Autodesk Inventor part; units mm, degrees
ref_plane "YZ Plane" through (0, 0, 0) normal (1, 0, 0) x (0, 1, 0)
ref_plane "XZ Plane" through (0, 0, 0) normal (0, 1, 0) x (-1, 0, 0)
ref_plane "XY Plane" through (0, 0, 0) normal (0, 0, 1) x (1, 0, 0)
sketch "Skizze3" plane through (0, 0, 0) normal (0, 1, 0) x (-1, 0, 0)
  line L0 (0, 0) -> (0, -150) construction
  line L1 (-10, 0) -> (-10, -150)
  line L2 (10, -150) -> (10, 0)
  arc A0 (10, 0) -> (-10, 0) centre (0, 0) ccw
  arc A1 (-10, -150) -> (10, -150) centre (0, -150) ccw
  circle A2 centre (0, 0) radius 5
  circle A3 centre (0, -150) radius 2.5
  circle A4 centre (0, -140) radius 1.5
  circle A5 centre (0, -115) radius 5
  circle A6 centre (0, -100) radius 5
  circle A7 centre (0, 0) radius 4.5
  circle A8 centre (0, -85) radius 5
  point P0 (0, -75)
  dimension "d4" = 150
  dimension "d5" = 10
  dimension "d6" = 10
  dimension "d7" = 5
  dimension "d8" = 3
  dimension "d9" = 10
  dimension "d12" = 10
  dimension "d13" = 10
  dimension "d15" = 15
  dimension "d27" = 9
  dimension "d34" = 115
  dimension "d35" = 15
extrude "Extrusion3" add sketch "Skizze3" along normal blind 5 contours A0 L2 A1 L1
sketch "Skizze4" plane through (0, 5, 0) normal (0, 1, 0) x (1, 0, 0)
  circle A0 centre (0, 0) radius 5
  circle A1 centre (0, 0) radius 10
  dimension "d18" = 20
extrude "Extrusion4" add sketch "Skizze4" along normal blind 5
extrude "Extrusion5" add sketch "Skizze3" along normal blind 6 contours A2
sketch "Skizze5" plane through (0, 0, 0) normal (0, -1, 0) x (1, 0, 0)
  circle A0 centre (0, -130) radius 5
  circle A1 centre (0, -100) radius 5
  circle A2 centre (0, -115) radius 5
  circle A3 centre (0, -100) radius 4.5
  circle A4 centre (0, -115) radius 4.5
  circle A5 centre (0, -130) radius 4.5
  point P0 (0, 0)
  point P1 (-1.5, -140)
  point P2 (-1.5, -140)
  dimension "d28" = 9
  dimension "d29" = 9
  dimension "d30" = 9
extrude "Extrusion7" add sketch "Skizze5" against normal blind 1 contours A1 | A2
equation "\"d4\" = Gelenk_Stifthalter"
equation "\"d35\" = d15"
equation "\"Gelenk_Stifthalter\" = 150"
properties part number "BT303_trajan20_21" material "Kunststoff, undurchsichtig Schwarz"
Can you work these out from the model? Positions are in its coordinate system, mm. A direction names the side the tool comes from. Give positions to 0.01 mm unless a question says otherwise; leave off trailing zeros. Order: outer loops, then holes, each group sorted by start corner. A loop starts at its lowest first (then second) coordinate and runs counter-clockwise, first axis right, second up. Notation, with made-up numbers: M 73.5,-7 L 131.5,-7 A22 cw 131.5,13 Z; hole C -7.75,-3 d10. An arc over 180 degrees is marked long. One line per item, written item: value.
Item 1: If we mould it in two halves opening along Z, with no side actions, what happens to faces 1 (the face through (0.195, 2.465, -141.487)), 2 (the face through (0, 2, -160)), 3 (the face through (10, 2, -74))? For each: pulls with the +Z half, pulls with the -Z half, needs draft (parallel to the pull), parting line crosses it, or undercut.
Verdict:
face 1: undercut
face 2: pulls with the -Z half
face 3: needs draft
Item 2: Please list where these lines run through material, in increasing order: line 1 (Z direction, x = -4, y = 2.5); line 2 (Z direction, x = 3, y = 1.75); line 3 (X direction, y = 3.2, z = -100).
Verdict:
line 1: -159.17 to -118, -112 to -103, -97 to -88, -82 to -2.06, 2.06 to 9.17
line 2: -159.54 to -119, -111 to -104, -96 to -89, -81 to -3.35, 3.35 to 9.54
line 3: -10 to -5, 5 to 10
Item 3: If we section it at B-B on y = 3: Write out the boundary of the cut face in (x, z).
Verdict:
outline: M -10,-150 A10 ccw 10,-150 L 10,0 A10 ccw -10,0 Z; hole C 0,-115 d10; hole C 0,-100 d10; hole C 0,-85 d10; hole C 0,0 d9; hole C 0,-150 d5; hole C 0,-140 d3
Item 4: For pin 1 (5 mm diameter, centred on x = -1, z = 2, fed in from +Y); pin 2 (11 mm diameter, centred on x = 2, z = -97.5, fed in from +Y), each with a flat end and sliding along its axis, tell me the tip position at first contact or that it passes through.
Verdict:
pin 1: y = 6
pin 2: y = 5
Item 5: If we section it at C-C on x = 0: State how many separate pieces and enclosed holes the cut face has, and give its area (3 significant figures).
Verdict:
separate pieces: 7
enclosed holes: 0
area: 668 mm2
Item 6: If we section it at D-D on z = -140: Write out the boundary of the cut face in (x, y).
Verdict:
outline: M -10,0 L -1.5,0 L -1.5,5 L -10,5 Z; M 1.5,0 L 10,0 L 10,5 L 1.5,5 Z
Item 7: For faces 4 (the face through (0, 0, -74)), 5 (the face through (1.08, 2.97, -110.12)), which set-ups out of +Z, -Z, +X, -X, +Y, -Y let a thin tool reach every point of the face, with its end or its side?
Verdict:
face 4: +Z, -Z, +X, -X, -Y
face 5: +Y
Item 8: If we section it at A-A on z = -100: Write out the boundary of the cut face in (x, y).
Verdict:
outline: M -10,0 L -4.5,0 L -4.5,1 L -5,1 L -5,5 L -10,5 Z; M 4.5,0 L 10,0 L 10,5 L 5,5 L 5,1 L 4.5,1 Z
